from build123d import *

# Parameters (mm, degrees)
CROQUIS1_R              = 8
CROQUIS1_R_2            = 0.76
SALIENTE_EXTRUIR1_DEPTH = 1.9
CORTAR_EXTRUIR1_START   = -10
CORTAR_EXTRUIR1_DEPTH   = 10
CROQUIS5_R              = 1.125
CORTAR_EXTRUIR2_DEPTH   = 52.936984895


with BuildPart() as part:
    # Croquis1 → Saliente-Extruir1 (new body)
    with BuildSketch(Plane(origin=(0, 0, 0), x_dir=(1, 0, 0), z_dir=(0, 1, 0))):
        with BuildLine():
            Line((16.42006532, 3.45), (29.59993468, 3.45))
            ThreePointArc((29.59993468, 3.45), (26.951107015, 7.365390191), (26.02, 12))
            Line((26.02, 12), (26.02, 13))
            ThreePointArc((26.02, 13), (29.241825407, 20.778174593), (37.02, 24))
            Line((37.02, 24), (46.02, 24))
            Line((46.02, 24), (46.02, 0))
            Line((46.02, 0), (30.96, 0))
            Line((30.96, 0), (30.96, -15))
            Line((30.96, -15), (15.06, -15))
            Line((15.06, -15), (15.06, 0))
            Line((15.06, 0), (0, 0))
            Line((0, 0), (0, 24))
            Line((0, 24), (9, 24))
            ThreePointArc((9, 24), (16.778174593, 20.778174593), (20, 13))
            Line((20, 13), (20, 12))
            ThreePointArc((20, 12), (19.068892985, 7.365390191), (16.42006532, 3.45))
        make_face()
        with Locations(Location((10, 14, 0), (0, 0, 90))):
            Circle(CROQUIS1_R, mode=Mode.SUBTRACT)
        with Locations(Location((1.67, 22.6, 0), (0, 0, 90))):
            Circle(CROQUIS1_R_2, mode=Mode.SUBTRACT)
        with Locations(Location((1.67, 5.4, 0), (0, 0, 90))):
            Circle(CROQUIS1_R_2, mode=Mode.SUBTRACT)
        with Locations(Location((36.02, 14, 0), (0, 0, 90))):
            Circle(CROQUIS1_R, mode=Mode.SUBTRACT)
        with Locations(Location((44.35, 5.4, 0), (0, 0, 90))):
            Circle(CROQUIS1_R_2, mode=Mode.SUBTRACT)
        with Locations(Location((44.35, 22.6, 0), (0, 0, 90))):
            Circle(CROQUIS1_R_2, mode=Mode.SUBTRACT)
    extrude(amount=SALIENTE_EXTRUIR1_DEPTH)

    # Croquis2 → Cortar-Extruir1 (cut)
    with BuildSketch(Plane(origin=(0, 1.9, 0), x_dir=(1, 0, 0), z_dir=(0, 1, 0)).offset(CORTAR_EXTRUIR1_START)):
        with BuildLine():
            Line((16.208454231, 24.753358164), (14, 20.92820323))
            ThreePointArc((14, 20.92820323), (18, 14), (14, 7.07179677))
            Line((14, 7.07179677), (16.208454231, 3.246641836))
            ThreePointArc((16.208454231, 3.246641836), (22.416908461, 14), (16.208454231, 24.753358164))
        make_face()
        with BuildLine():
            Line((32.02, 7.07179677), (29.811545769, 3.246641836))
            ThreePointArc((29.811545769, 3.246641836), (23.603091539, 14), (29.811545769, 24.753358164))
            Line((29.811545769, 24.753358164), (32.02, 20.92820323))
            ThreePointArc((32.02, 20.92820323), (28.02, 14), (32.02, 7.07179677))
        make_face()
    extrude(amount=CORTAR_EXTRUIR1_DEPTH, mode=Mode.SUBTRACT)

    # Croquis4 → Cortar-Revolución1 (revolve, cut)
    with BuildSketch(Plane.XY.offset(9)):
        with BuildLine():
            Line((22.51, 1.9), (23.51, 1.9))
            ThreePointArc((23.51, 1.9), (23.01, 1.4), (22.51, 1.9))
        make_face()
    revolve(axis=Axis((-976.99, 1.9, 9), (1, 0, 0)), mode=Mode.SUBTRACT)

    # Croquis5 → Cortar-Extruir2 (cut, through all)
    with BuildSketch(Plane(origin=(0, 1.9, 0), x_dir=(1, 0, 0), z_dir=(0, 1, 0))):
        with Locations(Location((23.01, -13, 0), (0, 0, 270))):
            Circle(CROQUIS5_R)
    extrude(amount=-CORTAR_EXTRUIR2_DEPTH, mode=Mode.SUBTRACT)


solid = part.part
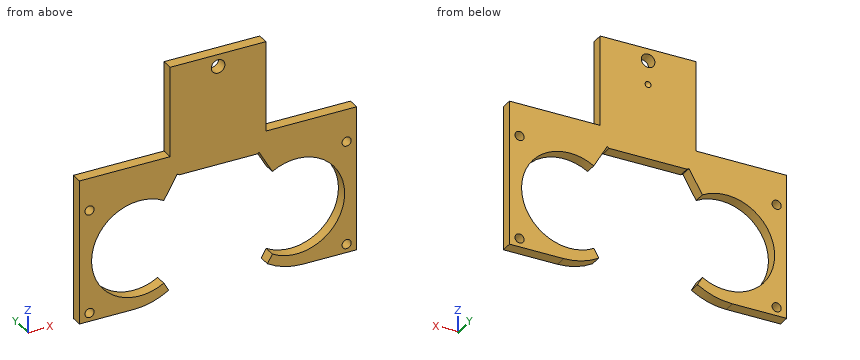
Read the model definition and answer for the solid it produces. Units are mm, in the model's axes. Coordinates: 2 decimals unless noted, no trailing zeros. Loops run counter-clockwise (first coordinate to the right, second up) from the corner with the lowest first, then second, coordinate; pieces in that order, holes last. Notation, with made-up numbers: (69.25, 64) -> (78.25, 64) arc R16 ccw to (78.25, 89) -> close; hole circle Ø3 at (-0.5, 50.5). An arc over 180 degrees is marked (long way). Answer in a Markdown table with one row per item.
Item 1: Straight lines are drawn through the part: line 1 along X through (y, z) = (1.05, -14); line 2 along X through (y, z) = (1.55, 7.5); line 3 along X through (y, z) = (0.25, -11). For each, find the intervals that lie inside material, in ascending order. Write a range as [from, to].
Returned:
| item | result |
|---|---|
| line 1 | x = [0, 2], [44.02, 46.02] |
| line 2 | x = [15.06, 30.96] |
| line 3 | x = [0, 2.58], [43.44, 46.02] |
Item 2: Each of these flat-tipped pins is pushed along its axis until it touches: P1, Ø0.6, axis at y = 0.5, z = 10, coming from the +X side; P2, Ø1, axis at x = 26, y = 1, coming from the -Z side. Where does it stop, or does it pass through?
Returned:
| item | result |
|---|---|
| P1 | stops at x = 30.96 |
| P2 | stops at z = -3.45 |
Item 3: A cutting plane is placed at A-A on z = -14. Determine the outline of the cut face in (x, y).
Returned:
| item | result |
|---|---|
| outline | (0, 0) -> (2, 0) -> (2, 1.9) -> (0, 1.9) -> close; (44.02, 0) -> (46.02, 0) -> (46.02, 1.9) -> (44.02, 1.9) -> close |
Item 4: A cutting plane is placed at C-C on y = 0.9. Determine the outline of the cut face in (x, z) (3 decimals).
Returned:
| item | result |
|---|---|
| outline | (0, -24) -> (9, -24) arc R11 ccw to (14.814, -22.338) -> (14, -20.928) arc R8 cw (long way) to (14, -7.072) -> (16.208, -3.247) arc R12.417 cw to (16.548, -3.45) -> (29.472, -3.45) arc R12.417 cw to (29.812, -3.247) -> (32.02, -7.072) arc R8 cw (long way) to (32.02, -20.928) -> (31.206, -22.338) arc R11 ccw to (37.02, -24) -> (46.02, -24) -> (46.02, 0) -> (30.96, 0) -> (30.96, 15) -> (15.06, 15) -> (15.06, 0) -> (0, 0) -> close; hole circle Ø1.52 at (1.67, -22.6); hole circle Ø1.52 at (1.67, -5.4); hole circle Ø2.25 at (23.01, 13); hole circle Ø1.52 at (44.35, -22.6); hole circle Ø1.52 at (44.35, -5.4) |
Item 5: A cutting plane is placed at D-D on z = 13. Determine the outline of the cut face in (x, y) (3 decimals).
Returned:
| item | result |
|---|---|
| outline | (15.06, 0) -> (21.885, 0) -> (21.885, 1.9) -> (15.06, 1.9) -> close; (24.135, 0) -> (30.96, 0) -> (30.96, 1.9) -> (24.135, 1.9) -> close |
Item 6: A cutting plane is placed at B-B on x = 23.01. Determine the outline of the cut face in (y, z) (3 decimals), plus the area to 3 significant figures.
Returned:
| item | result |
|---|---|
| outline | (0, -3.45) -> (1.9, -3.45) -> (1.9, 8.5) arc R0.5 cw to (1.9, 9.5) -> (1.9, 11.875) -> (0, 11.875) -> close; (0, 14.125) -> (1.9, 14.125) -> (1.9, 15) -> (0, 15) -> close |
| area | 30.4 mm^2 |
